The listing builds one solid part. Answer for the finished solid, in the listing's coordinates (mm). A direction names the side the tool comes from. Give positions to 0.01 mm unless a question says otherwise; leave off trailing zeros. Write each loop counter-clockwise with the first axis right and the second up, starting at its lowest first coordinate (ties: lowest second). Pieces come first, ordered by that corner, then holes. Notation, with made-up numbers: (56.25, 14) - (65.25, 14) arc R18 cw to (65.25, 40) - close; hole circle Ø3 at (-20.5, 31). An arc over 180 degrees is marked (long way). Return JSON: item names as keys, results as strings.
from build123d import *

# Parameters (mm, degrees)
SKETCH_1_R          = 4
EXTRUDE_1_DEPTH     = 3
SKETCH_3_R          = 4.6
EXTRUDE_2_DEPTH     = 0.6
EXTRUDE_START       = 0.6
SKETCH_4_R          = 4.6
EXTRUDE_3_DEPTH     = 0.6
SKETCH_5_R          = 1.75
CUT_EXTRUDE_1_DEPTH = 11


with BuildPart() as part:
    # 草图1 → 凸台-拉伸1 (new body)
    with BuildSketch(Plane(origin=(0, 0, 0), x_dir=(1, 0, 0), z_dir=(0, 1, 0))):
        with Locations(Location((0, 0, 0), (0, 0, 270))):
            Circle(SKETCH_1_R)
    extrude(amount=EXTRUDE_1_DEPTH)

    # 草图3 → 凸台-拉伸2 (add)
    with BuildSketch(Plane(origin=(0, 3, 0), x_dir=(1, 0, 0), z_dir=(0, 1, 0))):
        with Locations(Location((0, 0, 0), (0, 0, 270))):
            Circle(SKETCH_3_R)
    extrude(amount=EXTRUDE_2_DEPTH)

    # 草图4 → 凸台-拉伸3 (add)
    with BuildSketch(Plane.XZ.offset(EXTRUDE_START)):
        with Locations(Location((0, 0, 0), (0, 0, 90))):
            Circle(SKETCH_4_R)
    extrude(amount=-EXTRUDE_3_DEPTH)

    # 草图5 → 切除-拉伸1 (cut)
    with BuildSketch(Plane.XZ.offset(0.6)):
        with Locations(Location((0, 0, 0), (0, 0, 270))):
            Circle(SKETCH_5_R)
    extrude(amount=-CUT_EXTRUDE_1_DEPTH, mode=Mode.SUBTRACT)


solid = part.part
Item 1: A cutting plane is placed at D-D on y = 2.7. Determine the outline of the cut face in (x, z), then the cut area to 3 significant figures.
Answer below:
{"outline": "circle Ø8 at (0, 0); hole circle Ø3.5 at (0, 0)", "area": "40.6 mm²"}
Item 2: The mould has two halves that part along Y. Classify faces 1 (the face through (-3.8, 0, -1.7)), 2 (the face through (3.8, 3, -1.7)), 3 (the face through (0, -0.6, 2)), 4 (the face through (1.38, 3.3, 4.39)): +Y half, -Y half, draft (parallel to the pull), parting line (faces both ways), or undercut.
Answer below:
{"face 1": "undercut", "face 2": "undercut", "face 3": "-Y half", "face 4": "draft"}
Item 3: For faces 5 (the face through (-3.905, 1.479, -0.867)), 6 (the face through (0, 3.6, 2)), determine the directions among +Z, -Z, +X, -X, +Y, -Y from which every point of the face is accessible in a straight line to the end or side of a thin tool.
Answer below:
{"face 5": "none", "face 6": "+Z, -Z, +X, -X, +Y"}
Item 4: A cutting plane is placed at B-B on x = 0. Determine the outline of the cut face in (y, z).
Answer below:
{"outline": "(-0.6, -4.6) - (0, -4.6) - (0, -4) - (3, -4) - (3, -4.6) - (3.6, -4.6) - (3.6, -1.75) - (-0.6, -1.75) - close; (-0.6, 1.75) - (3.6, 1.75) - (3.6, 4.6) - (3, 4.6) - (3, 4) - (0, 4) - (0, 4.6) - (-0.6, 4.6) - close"}
Item 5: Consider L1, parallel to Y at x = 0.25, z = 4.25; L2, parallel to X at y = 0.35, z = 0; L3, parallel to Z at x = -1, y = 0.65. Determine where each line is inside the solid, lowest interval first.
Answer below:
{"L1": "y = -0.6 to 0, 3 to 3.6", "L2": "x = -4 to -1.75, 1.75 to 4", "L3": "z = -3.87 to -1.44, 1.44 to 3.87"}
Item 6: A cutting plane is placed at A-A on z = 0. Determine the outline of the cut face in (x, y).
Answer below:
{"outline": "(-4.6, -0.6) - (-1.75, -0.6) - (-1.75, 3.6) - (-4.6, 3.6) - (-4.6, 3) - (-4, 3) - (-4, 0) - (-4.6, 0) - close; (1.75, -0.6) - (4.6, -0.6) - (4.6, 0) - (4, 0) - (4, 3) - (4.6, 3) - (4.6, 3.6) - (1.75, 3.6) - close"}
Item 7: Flat-ended cylindrical pins translate along their axes: P1, Ø1.5, axis at x = -1.5, y = 0.5, coming from the -Z side; P2, Ø1, axis at x = -1.5, y = 3, coming from the +Z side. Find the tip coordinate at first contact, or state that the pin passes through.
Answer below:
{"P1": "stops at z = -4.5", "P2": "stops at z = 4.49"}
Item 8: A cutting plane is placed at C-C on x = 2.5. Determine the outline of the cut face in (y, z).
Answer below:
{"outline": "(-0.6, -3.86) - (0, -3.86) - (0, -3.12) - (3, -3.12) - (3, -3.86) - (3.6, -3.86) - (3.6, 3.86) - (3, 3.86) - (3, 3.12) - (0, 3.12) - (0, 3.86) - (-0.6, 3.86) - close"}
